Check sheet for the drawn part. Datum: minimum x, y, z corner. Units: mm. Coordinates: 2 decimals unless noted, no trailing zeros. Loops run counter-clockwise (first coordinate to the right, second up) from the corner with the lowest first, then second, coordinate; pieces in that order, holes last. Notation, with made-up numbers: (70, -25) - (95, -25) arc R5 ccw to (95, -16) - close; hole circle Ø10 at (57, 73). An arc over 180 degrees is marked (long way). Answer as a JSON object with one key per item and string values. Group by question number.
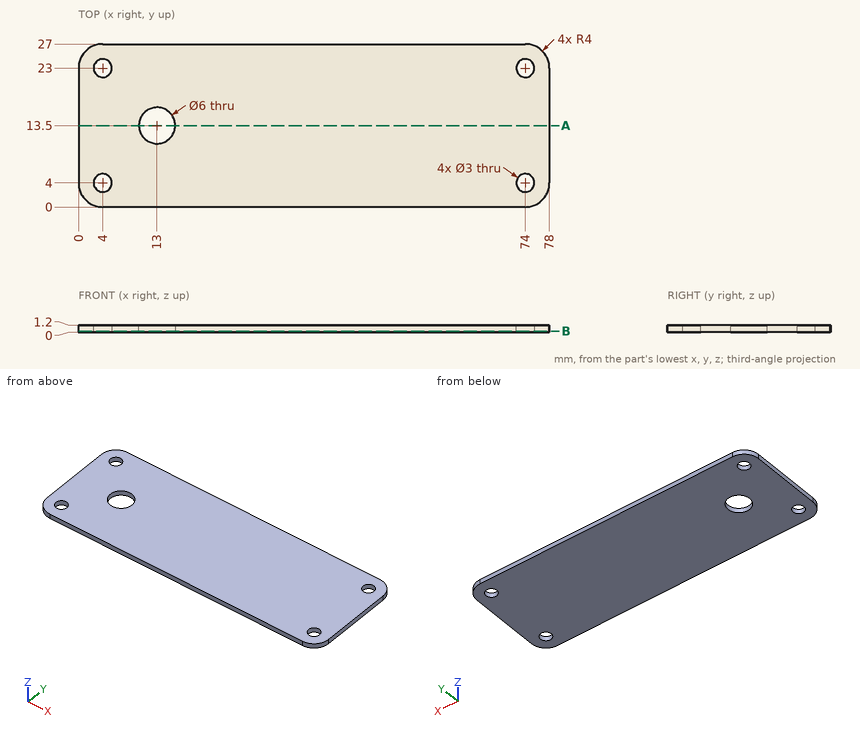
1. Sectioned sample at A-A on y = 13.5. Record the cut outline in (x, z).
2. Material ranges on line 1 (X direction, y = 23.25, z = 1.05); line 2 (X direction, y = 3, z = 0.5); line 3 (Y direction, x = 5, z = 1.15), recorded low to high.
3. Sectioned sample at B-B on z = 0.2. Record the cut outline in (x, y), plus the area to 3 significant figures.
Answers follow:
{
 "1": {"outline": "(0, 0) - (10, 0) - (10, 1.2) - (0, 1.2) - close; (16, 0) - (78, 0) - (78, 1.2) - (16, 1.2) - close"},
 "2": {"line 1": "x = 0.01 to 2.52, 5.48 to 72.52, 75.48 to 77.99", "line 2": "x = 0.13 to 2.88, 5.12 to 72.88, 75.12 to 77.87", "line 3": "y = 0 to 2.88, 5.12 to 21.88, 24.12 to 27"},
 "3": {"outline": "(0, 4) arc R4 ccw to (4, 0) - (74, 0) arc R4 ccw to (78, 4) - (78, 23) arc R4 ccw to (74, 27) - (4, 27) arc R4 ccw to (0, 23) - close; hole circle Ø3 at (4, 4); hole circle Ø3 at (4, 23); hole circle Ø6 at (13, 13.5); hole circle Ø3 at (74, 4); hole circle Ø3 at (74, 23)", "area": "2,040 mm^2"}
}
